Could you check a few things on this model? Use its own coordinates, in mm. Face numbers are marked on the shaded views. Coordinates: 2 decimals unless noted, no trailing zeros. Write each loop counter-clockwise with the first axis right and the second up, starting at its lowest first coordinate (ties: lowest second). Pieces come first, ordered by that corner, then holes.
Item 1: If I drill on probe 1 along Z at (x, y) = (-71, -56); probe 2 along Z at (x, y) = (-72, 104); probe 3 along Z at (x, y) = (-63, -33), over which ranges is the centre line in solid material (lowest first)?
Item 2: I want a section at C-C on z = 433.5. Please give me the cut outline in (x, y), then the cut area to 3 significant figures.
Item 3: For P1, Ø9.5, axis at y = -68, z = 468.5, coming from the +X side; P2, Ø14.5, axis at x = -78, y = -73, coming from the +Z side; P3, Ø4, axis at x = -57.5, y = 271, coming from the +Z side, each with a flat end and sliding along its axis, tell me the tip position at first contact or that it passes through.
Item 4: Thinking about a two-plate mould opening in Z: for the marked faces 1, 2 and 3, which applies, +Z half, -Z half, draft (parallel to the pull), parting line (faces both ways), or undercut?
Item 5: I want a section at A-A on y = 41. Please give me the cut outline in (x, z).
Item 6: I want a section at B-B on y = 211. Please give me the cut outline in (x, z), then the cut area to 3 significant figures.
from build123d import *

# Parameters (mm, degrees)
F0_W      = 10
F0_H      = 20
F1_DEPTH  = 10
F2_R      = 12
F3_DEPTH  = 450
F4_W      = 12
F4_H      = 12
F5_DEPTH  = 12
F6_W      = 38.0882956088
F6_H      = 12.0832407475
F7_DEPTH  = 10
F8_W      = 38.0462743342
F8_H      = 12.0327174664
F9_DEPTH  = 10
F10_R     = 12
F11_DEPTH = 225
F12_R     = 14
F13_DEPTH = 225


with BuildPart() as f1:
    # F0 (on Top) → F1 (new body)
    with BuildSketch(Plane.XY):
        Polygon((-96.8159428212, 10.2990681306), (-96.8159428212, -89.7009318694), (-46.8159428212, -89.7009318694), (-46.8159428212, 10.2990681306), (-56.8159428212, 10.2990681306), (-86.8159428212, 10.2990681306), align=None)
        with Locations((-91.8159428212, 20.2990681306)):
            Rectangle(F0_W, F0_H)
        Polygon((-86.8159428212, 30.2990681306), (-86.8159428212, 10.2990681306), (-56.8159428212, 10.2990681306), (-56.8159428212, 30.2990681306), (-56.8159428212, 50.2990681306), (-86.8159428212, 50.2990681306), align=None)
        with Locations((-51.8159428212, 20.2990681306)):
            Rectangle(F0_W, F0_H)
    extrude(amount=F1_DEPTH)

    # F2 (on face) → F3 (join)
    with BuildSketch(Plane.XY.offset(10)):
        with Locations((-71.8159428212, -70.8084776998)):
            Circle(F2_R)
    extrude(amount=F3_DEPTH)

    # F4 (on face) → F5 (join)
    with BuildSketch(Plane.XY.offset(460)):
        with Locations((-71.8180909753, -70.9205174615)):
            Rectangle(F4_W, F4_H)
    extrude(amount=F5_DEPTH)

    # F6 (on face) → F7 (join)
    with BuildSketch(Plane.YZ.offset(-65.8180909753)):
        with Locations((-69.3628769368, 466.0416203737)):
            Rectangle(F6_W, F6_H)
    extrude(amount=F7_DEPTH)

    # F8 (on face) → F9 (join)
    with BuildSketch(Plane(origin=(-77.8180909753, 0, 0), x_dir=(0, -1, 0), z_dir=(-1, 0, 0))):
        with Locations((69.303361699, 466.1028534174)):
            Rectangle(F8_W, F8_H)
    extrude(amount=F9_DEPTH)

    # F10 (on face) → F11 (join)
    with BuildSketch(Plane(origin=(0, -50.3187291324, 0), x_dir=(-1, 0, 0), z_dir=(0, 1, 0))):
        with Locations((71.529455483, 466.2147164345)):
            Circle(F10_R)
    extrude(amount=F11_DEPTH)

    # F12 (on face) → F13 (join)
    with BuildSketch(Plane(origin=(0, 174.6812708676, 0), x_dir=(-1, 0, 0), z_dir=(0, 1, 0))):
        with Locations((71.529455483, 466.2147164345)):
            Circle(F12_R)
    extrude(amount=F13_DEPTH)


solid = f1.part
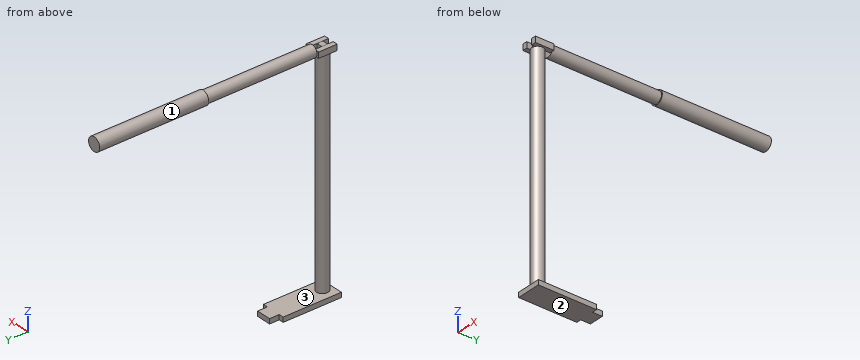
Response values:
1. probe 1: z = 0 to 10
1. probe 2: z = 454.22 to 478.21
1. probe 3: z = 0 to 10, 457.77 to 474.66
2. outline: circle Ø24 at (-71.82, -70.81)
2. area: 452 mm2
3. P1: stops at x = -55.82
3. P2: stops at z = 472.12
3. P3: stops at z = 473.38
4. face 1: parting line
4. face 2: -Z half
4. face 3: undercut
5. outline: (-86.82, 0) - (-56.82, 0) - (-56.82, 10) - (-86.82, 10) - close; circle Ø24 at (-71.53, 466.21)
6. outline: circle Ø28 at (-71.53, 466.21)
6. area: 616 mm2
